CAD build for the part. Positions are in the model's coordinates, mm. A direction names the side the tool comes from. Give positions to 0.01 mm unless a question says otherwise; leave off trailing zeros. Loops run counter-clockwise (first coordinate to the right, second up) from the corner with the lowest first, then second, coordinate; pieces in that order, holes last. Notation, with made-up numbers: M 37.5,25 L 71.5,25 A17 cw 71.5,30 Z; hole C -2.5,30 d2. An arc over 180 degrees is marked long. One line per question, with ' | ' between items.
```python
from build123d import *

# Parameters (mm, degrees)
F0_R     = 2
F1_DEPTH = 7.2
F3_DEPTH = 5.2
F4_R     = 2


# Not quite as in the source:
# - a fillet or chamfer that OpenCascade refuses, or shapes differently, is made with other operations: its cross-section is extruded or revolved along the edge and cut away or added
# - a feature names something its author has since deleted; it is built from what else it names


with BuildPart() as f1:
    # F0 (on Top) → F1 (new body)
    with BuildSketch(Plane.XY):
        with BuildLine():
            Line((-3.6799965084, -23), (39.5, -23))
            ThreePointArc((39.5, -23), (41.6213203436, -22.1213203436), (42.5, -20))
            Line((42.5, -20), (42.5, 20))
            ThreePointArc((42.5, 20), (41.6213203436, 22.1213203436), (39.5, 23))
            Line((39.5, 23), (-39.5, 23))
            ThreePointArc((-39.5, 23), (-41.6213203436, 22.1213203436), (-42.5, 20))
            Line((-42.5, 20), (-42.5, 0))
            Line((-42.5, 0), (-42.5, -20))
            ThreePointArc((-42.5, -20), (-41.6213203436, -22.1213203436), (-39.5, -23))
            Line((-39.5, -23), (-32.3200034916, -23))
            ThreePointArc((-32.3200034916, -23), (-31.4664395347, -22.8760091397), (-30.683431664, -22.5142857143))
            ThreePointArc((-30.683431664, -22.5142857143), (-18, -18.75), (-5.316568336, -22.5142857143))
            ThreePointArc((-5.316568336, -22.5142857143), (-4.5335604653, -22.8760091397), (-3.6799965084, -23))
        make_face()
        with Locations((-37.5, -18)):
            Circle(F0_R, mode=Mode.SUBTRACT)
        with Locations((37.5, -18)):
            Circle(F0_R, mode=Mode.SUBTRACT)
        with BuildLine():
            ThreePointArc((-31.75, 5.8896094947), (-18.5, 14.5), (-5.25, 5.8896094947))
            Line((-5.25, 5.8896094947), (-5.25, -5.8896094947))
            ThreePointArc((-5.25, -5.8896094947), (-18.5, -14.5), (-31.75, -5.8896094947))
            Line((-31.75, -5.8896094947), (-31.75, 5.8896094947))
        make_face(mode=Mode.SUBTRACT)
        with Locations((-37.5, 18)):
            Circle(F0_R, mode=Mode.SUBTRACT)
        with BuildLine():
            ThreePointArc((31.75, -5.8896094947), (18.5, -14.5), (5.25, -5.8896094947))
            Line((5.25, -5.8896094947), (5.25, 5.8896094947))
            ThreePointArc((5.25, 5.8896094947), (18.5, 14.5), (31.75, 5.8896094947))
            Line((31.75, 5.8896094947), (31.75, -5.8896094947))
        make_face(mode=Mode.SUBTRACT)
        with Locations((37.5, 18)):
            Circle(F0_R, mode=Mode.SUBTRACT)
    extrude(amount=F1_DEPTH)

    # F2 (on face) → F3 (cut)
    with BuildSketch(Plane(origin=(0, 0, 0), x_dir=(1, 0, 0), z_dir=(0, 0, -1))):
        with BuildLine():
            ThreePointArc((0, 4.2720018727), (-36.5, 0), (0, -4.2720018727))
            ThreePointArc((0, -4.2720018727), (36.5, 0), (0, 4.2720018727))
        make_face()
    extrude(amount=-F3_DEPTH, mode=Mode.SUBTRACT)

    # F4
    f4_edges = [f1.edges().sort_by_distance(p)[0] for p in [
        (0, 23, 7.2),
        (-41.62132, 22.12132, 7.2),
        (-42.5, 0, 7.2),
        (-41.62132, -22.12132, 7.2),
        (-35.910002, -23, 7.2),
        (17.910002, -23, 7.2),
        (41.62132, -22.12132, 7.2),
        (42.5, 0, 7.2),
        (41.62132, 22.12132, 7.2),
        (-18, -18.75, 7.2),
        (-31.46644, -22.876009, 7.2),
        (-4.53356, -22.876009, 7.2),
    ]]
    fillet(f4_edges, radius=F4_R)

    # F5: chamfer of 1.5 on 4 edges, made by hand

    # F5_s1 → F5_t2 (revolve, cut)
    with BuildSketch(Plane.XZ.offset(-18)):
        Polygon((-34, 7.2), (-35.5, 5.7), (-35.5, 7.2), align=None)
    revolve(axis=Axis((-37.5, 18, 7.2), (0, 0, 1)), mode=Mode.SUBTRACT)

    # F5_s3 → F5_t4 (revolve, cut)
    with BuildSketch(Plane.XZ.offset(18)):
        Polygon((-34, 7.2), (-35.5, 5.7), (-35.5, 7.2), align=None)
    revolve(axis=Axis((-37.5, -18, 7.2), (0, 0, 1)), mode=Mode.SUBTRACT)

    # F5_s5 → F5_t6 (revolve, cut)
    with BuildSketch(Plane.XZ.offset(18)):
        Polygon((41, 7.2), (39.5, 5.7), (39.5, 7.2), align=None)
    revolve(axis=Axis((37.5, -18, 7.2), (0, 0, 1)), mode=Mode.SUBTRACT)

    # F5_s7 → F5_t8 (revolve, cut)
    with BuildSketch(Plane.XZ.offset(-18)):
        Polygon((41, 7.2), (39.5, 5.7), (39.5, 7.2), align=None)
    revolve(axis=Axis((37.5, 18, 7.2), (0, 0, 1)), mode=Mode.SUBTRACT)


solid = f1.part
```
Item 1: Saw through at B-B on x = -18. Give the cut face in (y, z).
Conclusion:
outline: M -18.75,0 L -18.5,0 L -18.5,5.2 L -14.49,5.2 L -14.49,7.2 L -16.75,7.2 A2 ccw -18.75,5.2 Z; M 14.49,5.2 L 18.5,5.2 L 18.5,0 L 23,0 L 23,5.2 A2 ccw 21,7.2 L 14.49,7.2 Z
Item 2: Saw through at D-D on z = 1.25. Give the cut face in (x, y), and give its area (3 significant figures).
Conclusion:
outline: M -42.5,-20 A3 ccw -39.5,-23 L -32.32,-23 A3 ccw -30.68,-22.51 A23.25 cw -5.32,-22.51 A3 ccw -3.68,-23 L 39.5,-23 A3 ccw 42.5,-20 L 42.5,20 A3 ccw 39.5,23 L -39.5,23 A3 ccw -42.5,20 Z; hole C -37.5,-18 d4; hole C -37.5,18 d4; hole M 0,-4.27 A18.5 ccw long 0,4.27 A18.5 ccw long Z; hole C 37.5,-18 d4; hole C 37.5,18 d4 | area: 1,630 mm²
Item 3: Saw through at A-A on y = 0. Give the cut face in (x, z), and give its area (3 significant figures).
Conclusion:
outline: M -42.5,0 L -36.5,0 L -36.5,5.2 L -31.75,5.2 L -31.75,7.2 L -40.5,7.2 A2 ccw -42.5,5.2 Z; M -5.25,5.2 L 5.25,5.2 L 5.25,7.2 L -5.25,7.2 Z; M 31.75,5.2 L 36.5,5.2 L 36.5,0 L 42.5,0 L 42.5,5.2 A2 ccw 40.5,7.2 L 31.75,7.2 Z | area: 125 mm²
Item 4: 3-axis set-ups, long thin cutter, end or side, ignore diameter. For faces 1 (the flat face through (0, -1, 5.2)), 2 (the cylindrical face through (-31.48, -22.88, 2.56)), 3 (the flat face through (-5.25, 0, 6)): which of +Z, -Z, +X, -X, +Y, -Y reach the whole face in a straight line?
Conclusion:
face 1: -Z | face 2: +Z, -Z, -Y | face 3: +Z, -Z
Item 5: Mould opens along Y. For faces 4 (the cylindrical face through (-0.55, 22.4, 6.63)), 5 (the cylindrical face through (-36.485, -0.753, 2.564)), 6 (the cylindrical face through (-41.64, -22.1, 2.56)), 7 (the cylindrical face through (37.24, -16.017, 2.81)) say: pulls with the +Y half, pulls with the -Y half, needs draft (parallel to the pull), parting line crosses it, or undercut.
Conclusion:
face 4: pulls with the +Y half | face 5: undercut | face 6: pulls with the -Y half | face 7: undercut
Item 6: Drop flat-ended pins along their axis: P1, Ø2, axis at x = -7, z = 1, coming from the -Y side; P2, Ø1, axis at y = 2.5, z = 6, coming from the +X side; P3, Ø3.5, axis at x = -37.5, y = -18, coming from the +Z side. Give the stop position or say it passes through.
Conclusion:
P1: y = -22.09 | P2: x = 42.48 | P3: through
Item 7: Drill centre lines: line 1 along Y through (x, z) = (37.5, 1.45); line 2 along X through (y, z) = (19, 1.5); line 3 along Y through (x, z) = (-38, 0.5). Where is each one in solid material? Low to high. Write a range as [from, to].
Conclusion:
line 1: [-23, -20], [-16, 16], [20, 23] | line 2: [-42.5, -39.23], [-35.77, 35.77], [39.23, 42.5] | line 3: [-23, -19.94], [-16.06, 16.06], [19.94, 23]
Item 8: Saw through at C-C on x = -37.5. Give the cut face in (y, z).
Conclusion:
outline: M -23,0 L -20,0 L -20,5.7 L -21.45,7.15 A2 ccw -23,5.2 Z; M -16,0 L 16,0 L 16,5.7 L 14.5,7.2 L -14.5,7.2 L -16,5.7 Z; M 20,0 L 23,0 L 23,5.2 A2 ccw 21.45,7.15 L 20,5.7 Z
